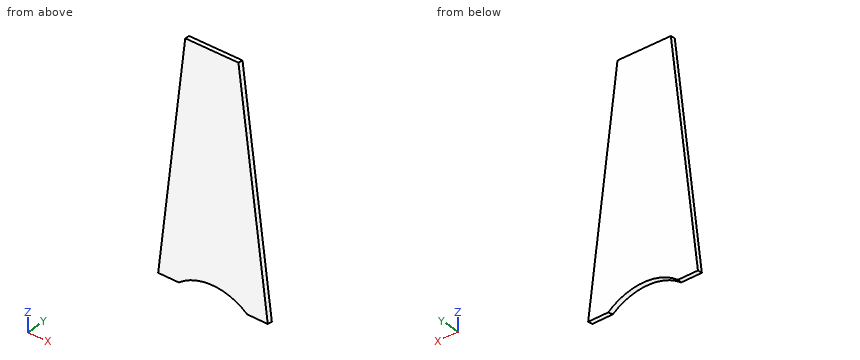
from build123d import *

# Parameters (mm, degrees)
F1_DEPTH = 19.05
F3_DEPTH = 19.05
F5_DEPTH = 419.1
F6_SIZE2 = 2.339036
F6_SIZE  = 19.04999


# Not quite as in the source:
# - a fillet or chamfer is up to 0.001 mm smaller than in the source, because OpenCascade refuses the exact size


with BuildPart() as f1:
    # F0 (on Front) → F1 (new body)
    with BuildSketch(Plane.XZ):
        Polygon((306.8257975104, 914.4), (103.6341967715, 912.5524640321), (0, 0), (419.1, 0), align=None)
    extrude(amount=F1_DEPTH)

    # F2 (on face) → F3 (cut)
    with BuildSketch(Plane.XZ.offset(19.05)):
        with BuildLine():
            Line((76.2, 0), (342.9, 0))
            ThreePointArc((342.9, 0), (209.55, 49.8767548608), (76.2, 0))
        make_face()
    extrude(amount=-F3_DEPTH, mode=Mode.SUBTRACT)

    # F4 (on Right) → F5 (cut)
    with BuildSketch(Plane.YZ):
        Polygon((-19.05, 2.3390458852), (-19.05, 0), (0, 0), align=None)
    extrude(amount=F5_DEPTH, mode=Mode.SUBTRACT)

    # F6 (size 19.05 and 2.3390458852 in the source; OpenCascade refuses exactly that, so slightly less here)
    f6_edges = [f1.edges().sort_by_distance(p)[0] for p in [
        (205.229997, 0, 913.476232),
    ]]
    f6_side = f1.faces().sort_by_distance((205.229997, -9.525, 913.476232))[0]
    chamfer(f6_edges, length=F6_SIZE, length2=F6_SIZE2, reference=f6_side)


solid = f1.part
Check sheet for the modelled part. Datum: model origin and axes. Units: mm. Give positions to 0.01 mm unless a question says otherwise; leave off trailing zeros. Loops run counter-clockwise (first coordinate to the right, second up) from the corner with the lowest first, then second, coordinate; pieces in that order, holes last. Notation, with made-up numbers: M 6.5,56 L 23.5,56 A28 ccw 23.5,74 Z; hole C 40.5,6.5 d10. An arc over 180 degrees is marked long. Answer as a JSON object with one key per item and string values. Group by question number.
Q1. Cross-section at A-A on y = -11.75. Record the cut outline in (x, z), then the cut area to 3 significant figures.
Q2. Cross-section at C-C on z = 483.5. Record the cut outline in (x, y), then the cut area to 3 significant figures.
Q3. Go/stop test with flat-tipped pins: P1, Ø1, axis at x = 72, y = -13.5, coming from the -Z side; P2, Ø1, axis at x = 300.5, y = -5.5, coming from the +Z side; P3, Ø8, axis at x = 157.5, y = -15, coming from the -Z side. Record where each tip stops, or that it passes through.
Q4. Material ranges on line 1 along X through (y, z) = (-0.75, 740); line 2 along X through (y, z) = (-11.5, 411); line 3 along Z through (x, y) = (216, -2), recorded low to high. Write a range as [from, to].
Evaluation:
{
 "1": {"outline": "M 0.16,1.44 L 77.88,1.44 A203.2 cw 341.22,1.44 L 418.92,1.44 L 306.94,913.5 L 103.53,911.66 Z", "area": "275,000 mm2"},
 "2": {"outline": "M 54.91,-19.05 L 359.73,-19.05 L 359.73,0 L 54.91,0 Z", "area": "5,810 mm2"},
 "3": {"P1": "stops at z = 1.6", "P2": "stops at z = 912.74", "P3": "stops at z = 41.99"},
 "4": {"line 1": "x = [84.04, 328.24]", "line 2": "x = [46.68, 368.64]", "line 3": "z = [49.77, 911.48]"}
}
